Autodesk Inventor part; units mm, degrees
ref_plane "YZ Plane" through (0, 0, 0) normal (1, 0, 0) x (0, 1, 0)
ref_plane "XZ Plane" through (0, 0, 0) normal (0, 1, 0) x (-1, 0, 0)
ref_plane "XY Plane" through (0, 0, 0) normal (0, 0, 1) x (1, 0, 0)
sketch "Sketch9" plane through (0, 0, 0) normal (0, 0, 1) x (1, 0, 0)
  line L0 (38.6921, -112.9498) -> (20.6921, -112.9498)
  arc A0 (18.6921, -110.9498) -> (20.6921, -112.9498) centre (20.6921, -110.9498) ccw
  line L1 (18.6921, -110.9498) -> (18.6921, -83.6655)
  line L2 (-0.9314, 4.1691) -> (18.6921, -83.6655)
  line L3 (-6.8342, 30.5897) -> (0, 0)
  arc A1 (-5.3184, 32.9777) -> (-6.8342, 30.5897) centre (-4.8823, 31.0258) ccw
  line L4 (12.2485, 36.9024) -> (-5.3184, 32.9777)
  line L5 (38.6921, -112.9498) -> (38.6921, -81.4586)
  line L6 (38.6921, -81.4586) -> (12.2485, 36.9024)
  point P0 (0, 0)
extrude "Extrusion8" add sketch "Sketch9" along normal mid plane 190
sketch "Sketch10" plane through (38.6921, -112.9498, 95) normal (1, 0, 0) x (0, 0, -1)
  point P0 (95, 112.9498)
sketch "Sketch11" plane through (0, 0, 0) normal (1, 0, 0) x (0, 1, 0)
  line L0 (-112.9498, 70) -> (-81.4586, 70)
  line L1 (-112.9498, -70) -> (-81.4586, -70)
  line L2 (-81.4586, -95) -> (-81.4586, 95)
  line L3 (-112.9498, 95) -> (-81.4586, 95)
  line L4 (-112.9498, -95) -> (-112.9498, 95)
  line L5 (-81.4586, -95) -> (-112.9498, -95)
  point P0 (0, 0)
  dimension "d39" = 140
  dimension "d40" = 70
extrude "Extrusion9" cut sketch "Sketch11" along normal through all both and the other way through all contours L4 L3 L2 L0 | L1 L2 L5 L4
sketch "Sketch12" plane through (12.2485, 36.9024, 95) normal (0.97594, 0.2180394, 0) x (0, 0, -1)
  line L0 (25, -121.279) -> (25, 0)
  line L1 (165, -121.279) -> (165, 0)
  line L2 (190, 0) -> (190, -121.279)
  line L3 (0, -121.279) -> (0, 0)
  line L4 (190, 0) -> (0, 0)
  line L5 (0, -121.279) -> (0, 0)
  line L6 (25, -121.279) -> (0, -121.279)
  line L7 (165, -121.279) -> (25, -121.279)
  line L8 (190, -121.279) -> (165, -121.279)
  line L9 (190, 0) -> (190, -121.279)
  point P0 (95, -33.3439)
  dimension "d44" = 25
  dimension "d45" = 25
  dimension "d46" = 140
extrude "Extrusion10" cut sketch "Sketch12" along normal through all both and the other way through all contours L6 L3 L4 L0 | L1 L4 L2 L8
sketch "Sketch13" plane through (12.2485, 36.9024, 70) normal (0.97594, 0.2180394, 0) x (0, 0, -1)
  line L0 (140, -152.0125) -> (0, -152.0125)
  line L1 (70, -152.0125) -> (70, -0.0751)
  circle A0 centre (115, -10.33) radius 3.4585
  circle A1 centre (25, -10.33) radius 3.4585
  circle A2 centre (-10, -105.33) radius 3.4585
  circle A3 centre (150, -105.33) radius 3.4585
  line L2 (0, 0) -> (140, 0)
  line L3 (0, 0) -> (0, -31.3439)
  line L4 (0, -31.3439) -> (12.5, -31.3439)
  line L5 (12.5, -31.3439) -> (12.5, -72.33)
  line L6 (12.5, -72.33) -> (0, -72.33)
  line L7 (0, -72.33) -> (0, -92.33)
  line L8 (-25, -92.33) -> (0, -92.33)
  ellipse E0 centre (2, -126.2447) end of major axis (2, -117.072) minor radius 2 (2, -117.072) -> (0.6988, -119.279) ccw
  line L9 (2, -117.072) -> (27.5, -117.072)
  line L10 (27.5, -27.072) -> (27.5, -117.072)
  line L11 (112.5, -27.072) -> (27.5, -27.072)
  line L12 (112.5, -117.072) -> (112.5, -27.072)
  line L13 (112.5, -117.072) -> (138, -117.072)
  ellipse E1 centre (138, -126.2447) end of major axis (138, -135.4173) minor radius 2 (139.3012, -119.279) -> (138, -117.072) ccw
  line L14 (165, -92.33) -> (165, -114.8107)
  line L15 (140, -92.33) -> (165, -92.33)
  line L16 (140, -92.33) -> (140, -72.33)
  line L17 (140, -72.33) -> (127.5, -72.33)
  line L18 (127.5, -72.33) -> (127.5, -31.3439)
  line L19 (127.5, -31.3439) -> (140, -31.3439)
  line L20 (140, -31.3439) -> (140, 0)
  line L21 (0, 0) -> (0, -121.279)
  line L22 (140, -121.279) -> (140, 0)
  line L23 (0, -121.279) -> (0, -152.0125)
  line L24 (0, -121.279) -> (-25, -121.279)
  line L25 (-25, -92.33) -> (-25, -121.279)
  line L26 (-25, -92.33) -> (7.4202, -92.33) construction
  line L27 (140, -121.279) -> (165, -121.279)
  line L28 (165, -92.33) -> (165, -121.279)
  point P0 (70, -33.3439)
  point P1 (-25.1048, -117.072)
  point P2 (-25, -119.279)
  point P3 (165, -119.279)
  dimension "d58" = 90
extrude "Extrusion11" add sketch "Sketch13" against normal up to surface (20 mm away) contours A2 | A3 | L8 L21 L24 L25 | L14 L28 L27 L22 L15
hole "Hole1" at (35.2146, -65.8933, -80) at (14.5009, 26.8209, -45) at (14.5009, 26.8209, 45) at (35.2146, -65.8933, 80) direction (-0.97594, -0.2180394, 0) diameter 6.917 depth 27.125 tip angle 118 counterbore diameter 10.025 counterbore depth 6.025
fillet "Fillet3" radius 5 2 edges at (35.5361, -67.3324, 95) (35.5361, -67.3324, -95)
properties part number "Cover of robot upper base" material "Steel, Alloy"
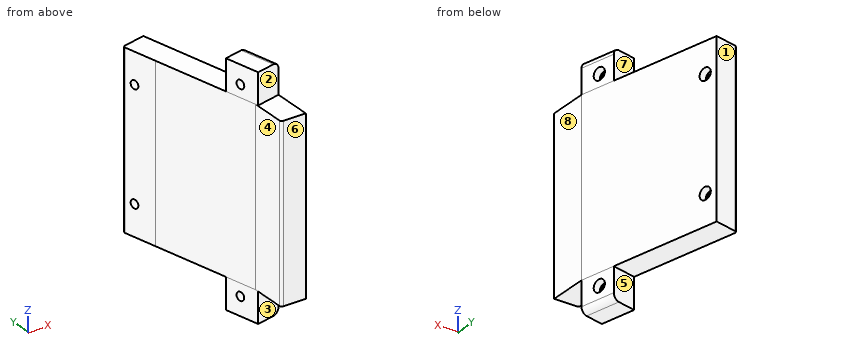
Design review of the part built by this model. Coordinates are the model's own, in mm. Face numbers are marked on the shaded views. A direction names the side the tool comes from. Round coordinates to 2 decimals unless told otherwise and drop trailing zeros. Order: outer loops, then holes, each group sorted by start corner. A loop starts at its lowest first (then second) coordinate and runs counter-clockwise, first axis right, second up. Notation, with made-up numbers: M -12,19.25 L 36,19.25 A13 ccw 36,40.25 Z; hole C 67.5,4 d5. An arc over 180 degrees is marked long. Put each result on its own line as item: value.
Q1. Draft analysis for pull direction Y (two halves, no side actions). For the marked faces 6, 7 and 8, state which applies: released by +Y, released by -Y, zero draft, split by the parting line, or undercut.
Reported:
face 6: released by -Y
face 7: released by +Y
face 8: zero draft
Q2. Consider section C-C (y = 8). State the section outline as (x, z) points.
Reported:
outline: M -1.79,-70 L 18.71,-70 L 18.71,70 L -1.79,70 Z
Q3. To check wall thickness, follow line 1 (Z direction, x = 4.5, y = 22.5); line 2 (Z direction, x = 19, y = -95.5); line 3 (Z direction, x = 9, y = 26.5). State the ranges of each line that lie inside material, in increasing order.
Reported:
line 1: -70 to -47.8, -42.2 to 42.2, 47.8 to 70
line 2: -70 to 70
line 3: -70 to -49.93, -40.07 to 40.07, 49.93 to 70
Q4. Insertion check: pin 1 Ø10 at (x, y) = (27.5, -101.5) entering from +Z; pin 2 Ø8 at (y, z) = (-98.5, 15.5) entering from -X; pin 3 Ø22 at (x, y) = (24, -98.5) entering from -Z. Each pin has a flat end and moves straight along its axis. Give the tip position at first contact, or say it passes through.
Reported:
pin 1: z = 70
pin 2: x = 18.69
pin 3: z = -70
Q5. Consider section B-B (y = -24). State the section outline as (x, z) points (3 decimals), and give its area (3 significant figures).
Reported:
outline: M 5.362,-70 L 25.855,-70 L 25.855,70 L 5.362,70 Z
area: 2,870 mm²
Q6. Machinability: for the marked faces 1, 2, 3, 4 and 5, which of the approach directions +Z, -Z, +X, -X, +Y, -Y give a long, thin tool a straight path to every point of the face, cutting with its end or side? Answer none if there is none.
Reported:
face 1: +Z, -Z, -X, +Y
face 2: +Z, +X, -Y
face 3: -Z, +X, -Y
face 4: +Z, -Z, -X, -Y
face 5: -Z, -X, +Y
Q7. Consider section A-A (z = 61.5). State the section outline as (x, y) points.
Reported:
outline: M -6.83,30.59 L -0.93,4.17 L 18.69,-83.67 L 18.69,-110.95 A2 ccw 20.69,-112.95 L 38.69,-112.95 L 38.69,-81.46 L 12.25,36.9 L -5.32,32.98 A2 ccw Z
